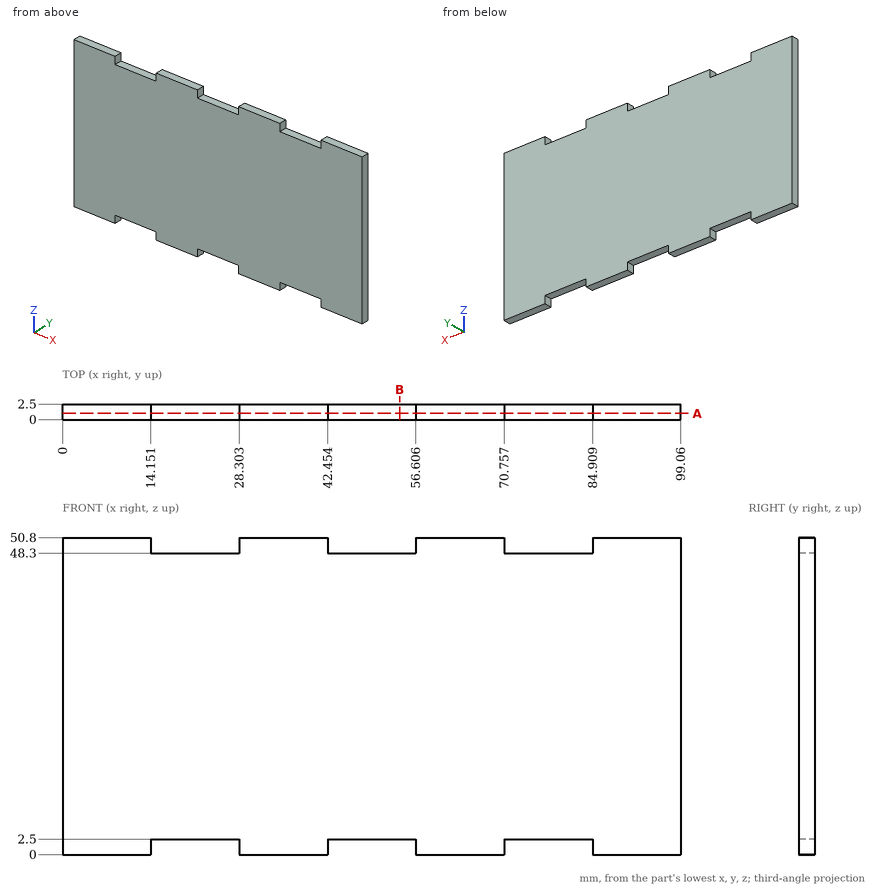
Geometry: see drawing. Coordinates: mm, zero at the bounding-box minimum. Round coordinates to 2 decimals unless told otherwise and drop trailing zeros. Order: outer loops, then holes, each group sorted by start corner. A loop starts at its lowest first (then second) coordinate and runs counter-clockwise, first axis right, second up. Notation, with made-up numbers: (-22.75, 42.25) -> (22.25, 42.25) arc R32 cw to (22.25, 75.25) -> close; hole circle Ø10 at (59, 10.25). An arc over 180 degrees is marked (long way). Write each question's results on one line, items separated by ' | '.
Q1. Section query A-A (y = 1). Output: boundary loops of the cut face in (x, z) (1 decimal).
Response values:
outline: (0, 0) -> (14.2, 0) -> (14.2, 2.5) -> (28.3, 2.5) -> (28.3, 0) -> (42.5, 0) -> (42.5, 2.5) -> (56.6, 2.5) -> (56.6, 0) -> (70.8, 0) -> (70.8, 2.5) -> (84.9, 2.5) -> (84.9, 0) -> (99.1, 0) -> (99.1, 50.8) -> (84.9, 50.8) -> (84.9, 48.3) -> (70.8, 48.3) -> (70.8, 50.8) -> (56.6, 50.8) -> (56.6, 48.3) -> (42.5, 48.3) -> (42.5, 50.8) -> (28.3, 50.8) -> (28.3, 48.3) -> (14.2, 48.3) -> (14.2, 50.8) -> (0, 50.8) -> close
Q2. Ray query, line 1 along Z through (x, y) = (21, 2.35). Return the intervals inside material, ascending.
Response values:
line 1: 2.5 to 48.3
Q3. Section query B-B (x = 54). Output: boundary loops of the cut face in (y, z).
Response values:
outline: (0, 2.5) -> (2.5, 2.5) -> (2.5, 48.3) -> (0, 48.3) -> close
Q4. Pin query (flat end, axial travel): pin 1 Ø0.8 at (x, y) = (18, 1) entering from +Z; pin 2 Ø1.2 at (x, y) = (23, 0.5) entering from -Z. Return the tip coordinate at first contact, or that it passes through.
Response values:
pin 1: z = 48.3 | pin 2: z = 2.5
